Work out the finished part from the listing and answer in its coordinate system (mm). A direction names the side the tool comes from. Coordinates: 2 decimals unless noted, no trailing zeros. Order: outer loops, then holes, each group sorted by start corner. A loop starts at its lowest first (then second) coordinate and runs counter-clockwise, first axis right, second up. Notation, with made-up numbers: (48.5, 51.5) -> (77.5, 51.5) arc R23 cw to (77.5, 77.5) -> close; hole circle Ø2 at (88, 17). An arc over 180 degrees is marked (long way). Use one line per item in the form item = value.
from build123d import *

# Parameters (mm, degrees)
SKETCH1_R           = 20
BOSS_EXTRUDE1_DEPTH = 15
SKETCH2_R           = 13
CUT_EXTRUDE1_DEPTH  = 10
SKETCH3_R           = 6
CUT_EXTRUDE2_DEPTH  = 5
SKETCH4_R           = 1.5
CUT_EXTRUDE3_DEPTH  = 15


with BuildPart() as part:
    # Sketch1 → Boss-Extrude1 (new body)
    with BuildSketch(Plane(origin=(0, 0, 0), x_dir=(1, 0, 0), z_dir=(0, 1, 0))):
        Circle(SKETCH1_R)
    extrude(amount=BOSS_EXTRUDE1_DEPTH)

    # Sketch2 → Cut-Extrude1 (cut)
    with BuildSketch(Plane(origin=(0, 15, 0), x_dir=(1, 0, 0), z_dir=(0, 1, 0))):
        Circle(SKETCH2_R)
    extrude(amount=-CUT_EXTRUDE1_DEPTH, mode=Mode.SUBTRACT)

    # Sketch3 → Cut-Extrude2 (cut)
    with BuildSketch(Plane(origin=(0, 5, 0), x_dir=(1, 0, 0), z_dir=(0, 1, 0))):
        Circle(SKETCH3_R)
    extrude(amount=-CUT_EXTRUDE2_DEPTH, mode=Mode.SUBTRACT)

    # Sketch4 → Cut-Extrude3 (cut)
    with BuildSketch(Plane(origin=(0, 15, 0), x_dir=(1, 0, 0), z_dir=(0, 1, 0))):
        with Locations((-10.493132047, -12.733584721)):
            Circle(SKETCH4_R)
        with Locations((-16.274173873, 2.720526557)):
            Circle(SKETCH4_R)
        with Locations((-5.781041827, 15.454111278)):
            Circle(SKETCH4_R)
        with Locations((10.493132047, 12.733584721)):
            Circle(SKETCH4_R)
        with Locations((16.274173873, -2.720526557)):
            Circle(SKETCH4_R)
        with Locations((5.781041827, -15.454111278)):
            Circle(SKETCH4_R)
    extrude(amount=-CUT_EXTRUDE3_DEPTH, mode=Mode.SUBTRACT)


solid = part.part
(1) Section D-D on y = 13.25 is taken. Write down the section's boundary in (x, z).
Data:
outline = circle Ø40 at (0, 0); hole circle Ø3 at (-16.27, -2.72); hole circle Ø26 at (0, 0); hole circle Ø3 at (-10.49, 12.73); hole circle Ø3 at (-5.78, -15.45); hole circle Ø3 at (5.78, 15.45); hole circle Ø3 at (10.49, -12.73); hole circle Ø3 at (16.27, 2.72)
(2) Which of the six approach directions +Z, -Z, +X, -X, +Y, -Y give full straight-line access (tool end or side, diameter ignored) to faces 4 (the cylindrical face through (11.3, 7.6, -14)), 5 (the cylindrical face through (-10.316, 10.07, 7.91))?
Data:
face_4 = +Y, -Y
face_5 = +Y
(3) Each of these flat-tipped pins is pushed along its axis until it touches: P1, Ø2.5, axis at x = 10.49, z = -12.73, coming from the -Y side; P2, Ø8, axis at y = 4.5, z = 15, coming from the +X side; P3, Ø1.5, axis at x = -8.5, y = 10.5, coming from the +Z side; P4, Ø1.5, axis at x = 11.5, y = 10, coming from the -Z side. Where does it stop, or does it pass through?
Data:
P1 = through
P2 = 16.7
P3 = 18.44
P4 = -16.87
(4) The mould has two halves that part along Z. Classify faces 1 (the cylindrical face through (-4.336, 7.395, 19.524)), 2 (the flat face through (13, 15, 4)), 3 (the flat face through (6, 5, 3)): released by +Z, released by -Z, zero draft, split by the parting line, or undercut.
Data:
face_1 = split by the parting line
face_2 = zero draft
face_3 = undercut
(5) Section C-C on x = -5.5 is taken. Write down the section's boundary in (y, z), plus the area to 3 significant figures.
Data:
outline = (0, -19.23) -> (15, -19.23) -> (15, -16.93) -> (0, -16.93) -> close; (0, -13.98) -> (15, -13.98) -> (15, -11.78) -> (5, -11.78) -> (5, -2.4) -> (0, -2.4) -> close; (0, 2.4) -> (5, 2.4) -> (5, 11.78) -> (15, 11.78) -> (15, 19.23) -> (0, 19.23) -> close
area = 273 mm²
(6) Straight lines are drawn through the part: line 1 along Z through (x, y) = (0, 9.5); line 2 along Z through (x, y) = (0, 1.1); line 3 along Z through (x, y) = (-6, 5.75). For each, find the intervals that lie inside material, in ascending order.
Data:
line_1 = -20 to -13, 13 to 20
line_2 = -20 to -6, 6 to 20
line_3 = -19.08 to -16.94, -13.97 to -11.53, 11.53 to 19.08
(7) Section B-B on z = 0 is taken. Write down the section's boundary in (x, y).
Data:
outline = (-20, 0) -> (-6, 0) -> (-6, 5) -> (-13, 5) -> (-13, 15) -> (-20, 15) -> close; (6, 0) -> (20, 0) -> (20, 15) -> (13, 15) -> (13, 5) -> (6, 5) -> close
(8) Section A-A on x = 0 is taken. Write down the section's boundary in (y, z).
Data:
outline = (0, -20) -> (15, -20) -> (15, -13) -> (5, -13) -> (5, -6) -> (0, -6) -> close; (0, 6) -> (5, 6) -> (5, 13) -> (15, 13) -> (15, 20) -> (0, 20) -> close
